Part model, mm, in its own coordinate system. A direction names the side the tool comes from. Round coordinates to 2 decimals unless told otherwise and drop trailing zeros. Loops run counter-clockwise (first coordinate to the right, second up) from the corner with the lowest first, then second, coordinate; pieces in that order, holes last.
from build123d import *

# Parameters (mm, degrees)
SKETCH_1_W           = 25
SKETCH_1_H           = 25
SKETCH_1_W_2         = 13
SKETCH_1_H_2         = 13
EXTRUDE_1_DEPTH      = 4
EXTRUDE_5_DEPTH      = 4
EXTRUDE_5_DEPTH_BACK = 4
EXTRUDE_6_DEPTH      = 8
EXTRUDE_7_DEPTH      = 8
SKETCH_10_W          = 13
SKETCH_10_H          = 13.001688454
EXTRUDE_8_DEPTH      = 2
SKETCH_11_R          = 1.25
CUT_EXTRUDE_1_DEPTH  = 54.272882407


with BuildPart() as part:
    # Эскиз1 → Бобышка-Вытянуть1 (new body)
    with BuildSketch(Plane(origin=(0, 0, 0), x_dir=(1, 0, 0), z_dir=(0, 1, 0))):
        with Locations((6.5, 6.5)):
            Rectangle(SKETCH_1_W, SKETCH_1_H)
        with Locations((6.5, 6.5)):
            Rectangle(SKETCH_1_W_2, SKETCH_1_H_2, mode=Mode.SUBTRACT)
    extrude(amount=EXTRUDE_1_DEPTH)

    # Эскиз6 → Бобышка-Вытянуть5 (add, two sides: drawn at the far end of the back side and taken through both)
    with BuildSketch(Plane(origin=(0, 0, -6.5), x_dir=(-1, 0, 0), z_dir=(0, 0, -1)).offset(-EXTRUDE_5_DEPTH_BACK)):
        Polygon((-13, 4), (-9, 4), (-9, -40), (-6, -40), (-6, -42), (-11, -42), (-11, 2), (-13, 2), align=None)
    extrude(amount=EXTRUDE_5_DEPTH + EXTRUDE_5_DEPTH_BACK)

    # Эскиз7 → Бобышка-Вытянуть6 (add)
    with BuildSketch(Plane(origin=(0, 0, -10.5), x_dir=(-1, 0, 0), z_dir=(0, 0, -1))):
        Polygon((-9, -40), (-9, 4), (-6, -40), align=None)
    extrude(amount=-EXTRUDE_6_DEPTH)

    # Эскиз9 → Бобышка-Вытянуть7 (add)
    with BuildSketch(Plane.XY.offset(-2.5)):
        with BuildLine():
            Line((9, 4), (0, 4))
            Line((0, 4), (0, 2))
            ThreePointArc((0, 2), (6.069824399, -2.94312486), (8.009524283, -10.526977177))
            Line((8.009524283, -10.526977177), (9, 4))
        make_face()
    extrude(amount=-EXTRUDE_7_DEPTH)

    # Эскиз10 → Бобышка-Вытянуть8 (add)
    with BuildSketch(Plane(origin=(0, 4, 0), x_dir=(1, 0, 0), z_dir=(0, 1, 0))):
        with Locations((6.5, 6.499155773)):
            Rectangle(SKETCH_10_W, SKETCH_10_H)
    extrude(amount=-EXTRUDE_8_DEPTH)

    # Эскиз11 → Вырез-Вытянуть1 (cut, through all)
    with BuildSketch(Plane(origin=(0, 4, 0), x_dir=(1, 0, 0), z_dir=(0, 1, 0))):
        with Locations(Location((-2.5, 15.5, 0), (0, 0, 270))):
            Circle(SKETCH_11_R)
        with Locations(Location((15.5, 15.5, 0), (0, 0, 270))):
            Circle(SKETCH_11_R)
        with Locations(Location((-2.5, -2.5, 0), (0, 0, 270))):
            Circle(SKETCH_11_R)
        with Locations(Location((15.5, -2.5, 0), (0, 0, 270))):
            Circle(SKETCH_11_R)
    extrude(amount=-CUT_EXTRUDE_1_DEPTH, mode=Mode.SUBTRACT)


solid = part.part
1) Tool access for faces 1 (the face through (-2.45, 2.03, -16.75)), 2 (the face through (19, 2, -6)), 3 (the face through (6.01, -2.85, -6.44)), 4 (the face through (6, 1, -13)), 5 (the face through (7.02, -25.06, -6.56)): list every direction of +Z, -Z, +X, -X, +Y, -Y with a clear straight run to the whole face (end or side of a thin tool).
Values:
face 1: +Y, -Y
face 2: +Z, -Z, +X, +Y, -Y
face 3: none
face 4: -Y
face 5: +Z, -Z, -X
2) Slice it at D-D, the plane x = 16. Give the cut face in (y, z), then the cut area to 3 significant figures.
Values:
outline: (0, -19) - (4, -19) - (4, -16.65) - (0, -16.65) - close; (0, -14.35) - (4, -14.35) - (4, 1.35) - (0, 1.35) - close; (0, 3.65) - (4, 3.65) - (4, 6) - (0, 6) - close
area: 81.7 mm2
3) Mould opens along X. For faces 6 (the face through (6, 2, 6)), 7 (the face through (6, -41, -6)), 8 (the face through (6, 2, -2)) say: released by +X, released by -X, zero draft, split by the parting line, or undercut.
Values:
face 6: zero draft
face 7: released by -X
face 8: undercut
4) Slice it at B-B, the plane y = 0.5. Give the cut face in (x, z), then the cut area to 3 significant figures.
Values:
outline: (-6, -19) - (19, -19) - (19, 6) - (-6, 6) - close; (2.8, -10.5) - (11, -10.5) - (11, -2.5) - (2.8, -2.5) - close; hole circle Ø2.5 at (-2.5, -15.5); hole circle Ø2.5 at (-2.5, 2.5); hole (0, -13) - (13, -13) - (13, 0) - (0, 0) - close; hole circle Ø2.5 at (15.5, -15.5); hole circle Ø2.5 at (15.5, 2.5)
area: 502 mm2
5) Slice it at A-A, the plane z = 2.5. Give the cut face in (x, y).
Values:
outline: (-6, 0) - (-3.75, 0) - (-3.75, 4) - (-6, 4) - close; (-1.25, 0) - (14.25, 0) - (14.25, 4) - (-1.25, 4) - close; (16.75, 0) - (19, 0) - (19, 4) - (16.75, 4) - close
6) Drop flat-ended pins along their axis: pin 1 Ø6 at (x, y) = (9.5, -4) entering from +Z; pin 2 Ø1.5 at (x, z) = (15.5, -15.5) entering from +Y; pin 3 Ø5.5 at (x, y) = (7.5, -10) entering from -Z; pin 4 Ø2 at (y, z) = (-41, -5) entering from -X. Give the stop position or say it passes through.
Values:
pin 1: stops at z = -2.5
pin 2: passes through
pin 3: stops at z = -10.5
pin 4: stops at x = 6
7) Slice it at C-C, the plane x = 9.25. Give the cut face in (y, z).
Values:
outline: (-42, -10.5) - (2, -10.5) - (2, -13) - (0, -13) - (0, -19) - (4, -19) - (4, 6) - (0, 6) - (0, 0) - (2, 0) - (2, -2.5) - (-42, -2.5) - close
8) Wall check: line 1 along X through (y, z) = (2.6, -15.5); line 2 along X through (y, z) = (1.5, -1); line 3 along Y through (x, z) = (2, -13.75). Give the ranges that are in metal, low to high.
Values:
line 1: x = -6 to -3.75, -1.25 to 14.25, 16.75 to 19
line 2: x = -6 to 0, 13 to 19
line 3: y = 0 to 4
